Design review of the part built by this model. Coordinates are the model's own, in mm. Face numbers are marked on the shaded views. A direction names the side the tool comes from. Coordinates: 2 decimals unless noted, no trailing zeros. Order: outer loops, then holes, each group sorted by start corner. A loop starts at its lowest first (then second) coordinate and runs counter-clockwise, first axis right, second up. Notation, with made-up numbers: M 70,6 L 115,6 A19 cw 115,41 Z; hole C 49,-21 d9. An arc over 180 degrees is marked long. Answer in a Markdown table with one row per item.
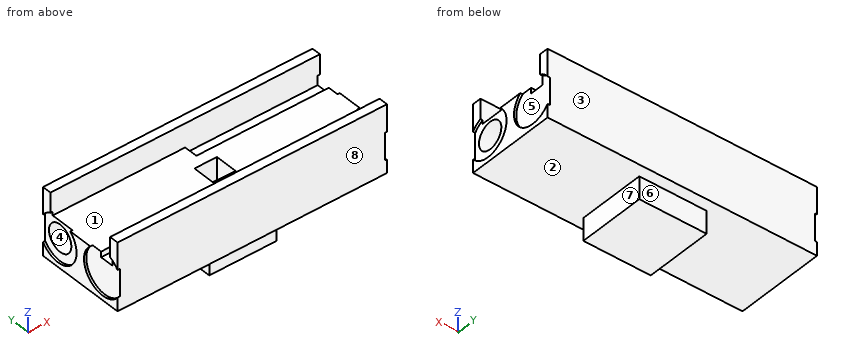
from build123d import *

# Parameters (mm, degrees)
SKETCH1_W           = 120
SKETCH1_H           = 40
BOSS_EXTRUDE1_DEPTH = 30
CUT_EXTRUDE1_DEPTH  = 60
CUT_EXTRUDE2_DEPTH  = 60
SKETCH6_W           = 30
SKETCH6_H           = 30
BOSS_EXTRUDE2_DEPTH = 10
SKETCH7_R           = 10
CUT_EXTRUDE3_DEPTH  = 1
SKETCH9_R           = 6
CUT_EXTRUDE4_DEPTH  = 35
SKETCH10_R          = 6
CUT_EXTRUDE5_DEPTH  = 35
SKETCH11_W          = 10
SKETCH11_H          = 10
CUT_EXTRUDE6_DEPTH  = 10


with BuildPart() as part:
    # Sketch1 → Boss-Extrude1 (new body)
    with BuildSketch(Plane.XY):
        with Locations((354.047582571, 83.912277662)):
            Rectangle(SKETCH1_W, SKETCH1_H)
    extrude(amount=BOSS_EXTRUDE1_DEPTH)

    # Sketch2 → Cut-Extrude1 (cut)
    with BuildSketch(Plane(origin=(414.047582571, 0, 0), x_dir=(0, 0, -1), z_dir=(1, 0, 0))):
        Polygon((-30, 99.912277662), (-19.5, 99.912277662), (-17, 99.912277662), (-17, 93.912277662), (-19.5, 93.912277662), (-19.5, 67.912277662), (-30, 67.912277662), align=None)
    extrude(amount=-CUT_EXTRUDE1_DEPTH, mode=Mode.SUBTRACT)

    # Sketch5 → Cut-Extrude2 (cut)
    with BuildSketch(Plane.ZY.offset(-294.047582571)):
        Polygon((30, 99.912277662), (19.5, 99.912277662), (19.5, 73.912277662), (17, 73.912277662), (17, 67.912277662), (19.5, 67.912277662), (30, 67.912277662), align=None)
    extrude(amount=-CUT_EXTRUDE2_DEPTH, mode=Mode.SUBTRACT)

    # Sketch6 → Boss-Extrude2 (add)
    with BuildSketch(Plane(origin=(0, 0, 0), x_dir=(-1, 0, 0), z_dir=(0, 0, -1))):
        with Locations((-354.047582571, 83.912277662)):
            Rectangle(SKETCH6_W, SKETCH6_H)
    extrude(amount=BOSS_EXTRUDE2_DEPTH)

    # Sketch7 → Cut-Extrude3 (cut)
    with BuildSketch(Plane(origin=(414.047582571, 0, 0), x_dir=(0, 0, -1), z_dir=(1, 0, 0))):
        with Locations((-12, 95.912277662)):
            Circle(SKETCH7_R)
        with Locations((-12, 71.912277662)):
            Circle(SKETCH7_R)
    cut_extrude3 = extrude(amount=-CUT_EXTRUDE3_DEPTH, mode=Mode.SUBTRACT)

    # Mirror1: Cut-Extrude3 across plane
    add(cut_extrude3.mirror(Plane.ZY.offset(-354.047582571)), mode=Mode.SUBTRACT)

    # Sketch9 → Cut-Extrude4 (cut)
    with BuildSketch(Plane(origin=(413.047582571, 0, 0), x_dir=(0, 0, -1), z_dir=(1, 0, 0))):
        with Locations((-12, 71.912277662)):
            Circle(SKETCH9_R)
    extrude(amount=-CUT_EXTRUDE4_DEPTH, mode=Mode.SUBTRACT)

    # Sketch10 → Cut-Extrude5 (cut)
    with BuildSketch(Plane.ZY.offset(-295.047582571)):
        with Locations((12, 95.912277662)):
            Circle(SKETCH10_R)
    extrude(amount=-CUT_EXTRUDE5_DEPTH, mode=Mode.SUBTRACT)

    # Sketch11 → Cut-Extrude6 (cut)
    with BuildSketch(Plane.XY.offset(19.5)):
        with Locations((354.047582571, 83.912277662)):
            Rectangle(SKETCH11_W, SKETCH11_H)
    extrude(amount=-CUT_EXTRUDE6_DEPTH, mode=Mode.SUBTRACT)


solid = part.part
(1) Add section C-C, the plane z = 12. Give the boundary of the cut face in (x, y), and give its area (3 significant figures).
Return value:
| item | result |
|---|---|
| outline | M 294.05,81.91 L 295.05,81.91 L 295.05,63.91 L 413.05,63.91 L 413.05,65.91 L 378.05,65.91 L 378.05,77.91 L 413.05,77.91 L 413.05,81.91 L 414.05,81.91 L 414.05,85.91 L 413.05,85.91 L 413.05,103.91 L 295.05,103.91 L 295.05,101.91 L 330.05,101.91 L 330.05,89.91 L 295.05,89.91 L 295.05,85.91 L 294.05,85.91 Z; hole M 349.05,78.91 L 359.05,78.91 L 359.05,88.91 L 349.05,88.91 Z |
| area | 3,790 mm2 |
(2) For the marked faces 4, 5, 6, 7 and 8, list the 3-axis set-ups (+Z, -Z, +X, -X, +Y, -Y) from which the entire face can be reached by the end or side of a thin tool; tool diameter is ignored.
Return value:
| item | result |
|---|---|
| face 4 | -X |
| face 5 | +X |
| face 6 | -Z, +X, -X, +Y |
| face 7 | -Z, +X, +Y, -Y |
| face 8 | +Z, -Z, +X, -X, -Y |
(3) Draft analysis for pull direction Y (two halves, no side actions). For the marked faces 1, 2 and 3, state which applies: pulls with the +Y half, pulls with the -Y half, needs draft (parallel to the pull), parting line crosses it, or undercut.
Return value:
| item | result |
|---|---|
| face 1 | undercut |
| face 2 | needs draft |
| face 3 | pulls with the +Y half |
(4) For line 1 along Y through (x, z) = (364, 18.5); line 2 along Y through (x, z) = (310, 25); line 3 along X through (y, z) = (91, 4.5), list the stretches that pass through material, from the lowest coordinate up. Write a range as from..to.
Return value:
| item | result |
|---|---|
| line 1 | y = 63.91..93.91, 99.91..103.91 |
| line 2 | y = 63.91..67.91, 99.91..103.91 |
| line 3 | x = 295.05..413.05 |
(5) Add section B-B, the plane x = 322. Give the boundary of the cut face in (y, z).
Return value:
| item | result |
|---|---|
| outline | M 63.91,0 L 103.91,0 L 103.91,30 L 99.91,30 L 99.91,19.5 L 73.91,19.5 L 73.91,17 L 67.91,17 L 67.91,30 L 63.91,30 Z; hole C 95.91,12 d12 |
(6) Add section A-A, the plane z = 27. Give the boundary of the cut face in (x, y).
Return value:
| item | result |
|---|---|
| outline | M 294.05,63.91 L 414.05,63.91 L 414.05,67.91 L 294.05,67.91 Z; M 294.05,99.91 L 414.05,99.91 L 414.05,103.91 L 294.05,103.91 Z |
(7) Insertion check: pin 1 Ø6 at (x, y) = (347, 80.5) entering from +Z; pin 2 Ø3.5 at (y, z) = (98, 9.5) entering from -X; pin 3 Ø1 at (y, z) = (95.5, 14) entering from +X; pin 4 Ø8 at (x, z) = (352, -3) entering from -Y. Each pin has a flat end and moves straight along its axis. Give the tip position at first contact, or say it passes through.
Return value:
| item | result |
|---|---|
| pin 1 | stops at z = 19.5 |
| pin 2 | stops at x = 330.05 |
| pin 3 | stops at x = 413.05 |
| pin 4 | stops at y = 63.91 |
(8) Add section D-D, the plane x = 351. Give the boundary of the cut face in (y, z).
Return value:
| item | result |
|---|---|
| outline | M 63.91,0 L 68.91,0 L 68.91,-10 L 98.91,-10 L 98.91,0 L 103.91,0 L 103.91,30 L 99.91,30 L 99.91,19.5 L 88.91,19.5 L 88.91,9.5 L 78.91,9.5 L 78.91,19.5 L 73.91,19.5 L 73.91,17 L 67.91,17 L 67.91,30 L 63.91,30 Z |
